Can you work these out from the drawing? Everything is in mm from the part's minimum corner. Coordinates: 2 decimals unless noted, no trailing zeros. Order: outer loops, then holes, each group sorted by start corner. A loop starts at its lowest first (then second) coordinate and runs counter-clockwise, first axis right, second up. Notation, with made-up numbers: (83, -11) -> (100, -11) arc R12 cw to (100, -6) -> close; hole circle Ø6 at (35, 25.25). An arc over 180 degrees is marked (long way). Return JSON: item names as keys, results as strings. Group by question number.
1) Thinking about a two-plate mould opening in X: for the marked faces 1, 2 and 3, which applies, +X half, -X half, draft (parallel to the pull), parting line (faces both ways), or undercut?
2) If I drill on probe 1 along Y at (x, z) = (7.5, 13) (3 decimals); probe 2 along X at (y, z) = (77.5, 18.75); probe 3 along Y at (x, z) = (9.75, 16.5), over which ranges is the centre line in solid material (lowest first)? Write a range as from..to.
3) If we section it at B-B, the plane z = 13.5: Please give me the cut outline in (x, y) (3 decimals).
4) If we section it at A-A, the plane x = 7.5: Please give me the cut outline in (y, z) (3 decimals).
5) If we section it at C-C, the plane y = 13.5: Please give me the cut outline in (x, z).
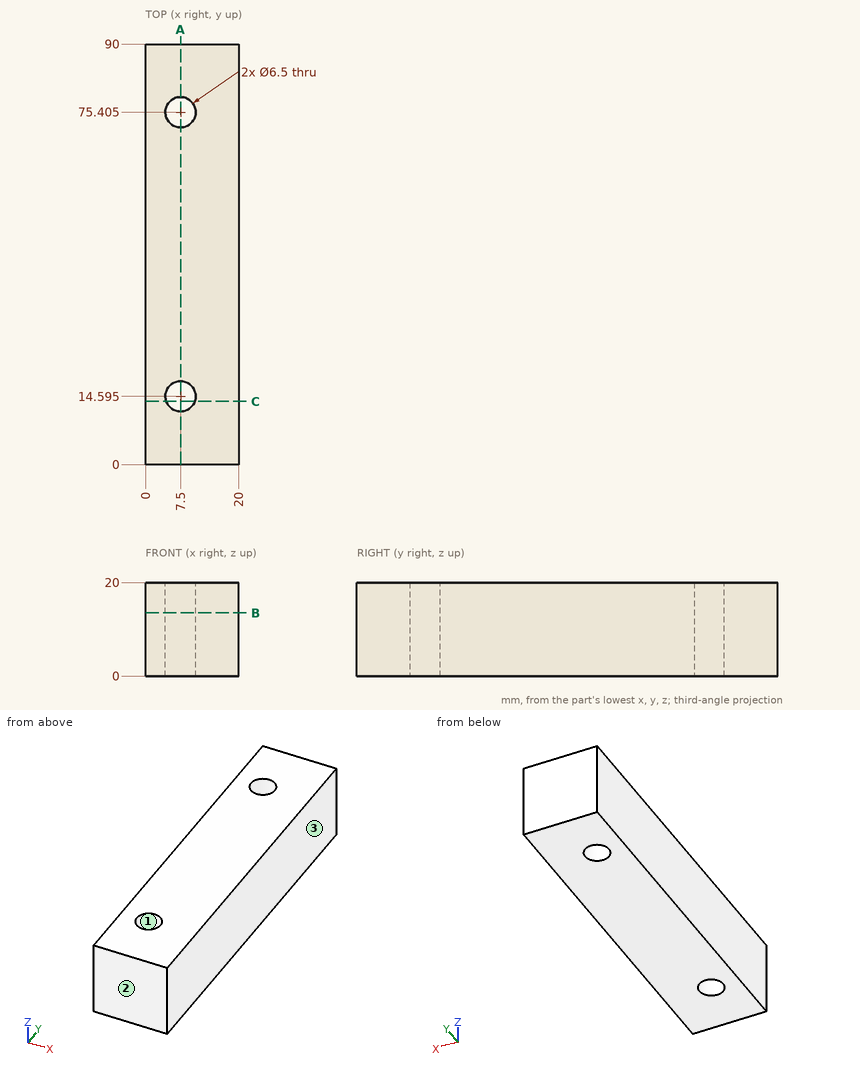
Result sheet:
{
 "1": {"face 1": "undercut", "face 2": "draft", "face 3": "+X half"},
 "2": {"probe 1": "y = 0..11.345, 17.845..72.155, 78.655..90", "probe 2": "x = 0..5.02, 9.98..20", "probe 3": "y = 0..12.25, 16.94..73.06, 77.75..90"},
 "3": {"outline": "(0, 0) -> (20, 0) -> (20, 90) -> (0, 90) -> close; hole circle Ø6.5 at (7.5, 14.595); hole circle Ø6.5 at (7.5, 75.405)"},
 "4": {"outline": "(0, 0) -> (11.345, 0) -> (11.345, 20) -> (0, 20) -> close; (17.845, 0) -> (72.155, 0) -> (72.155, 20) -> (17.845, 20) -> close; (78.655, 0) -> (90, 0) -> (90, 20) -> (78.655, 20) -> close"},
 "5": {"outline": "(0, 0) -> (4.44, 0) -> (4.44, 20) -> (0, 20) -> close; (10.56, 0) -> (20, 0) -> (20, 20) -> (10.56, 20) -> close"}
}
